Could you check a few things on this drawing? It's one solid part, dimensions in mm from its lowest x, y, z. Coordinates: 2 decimals unless noted, no trailing zeros. Order: outer loops, then holes, each group sorted by start corner. A loop starts at its lowest first (then second) coordinate and runs counter-clockwise, first axis right, second up.
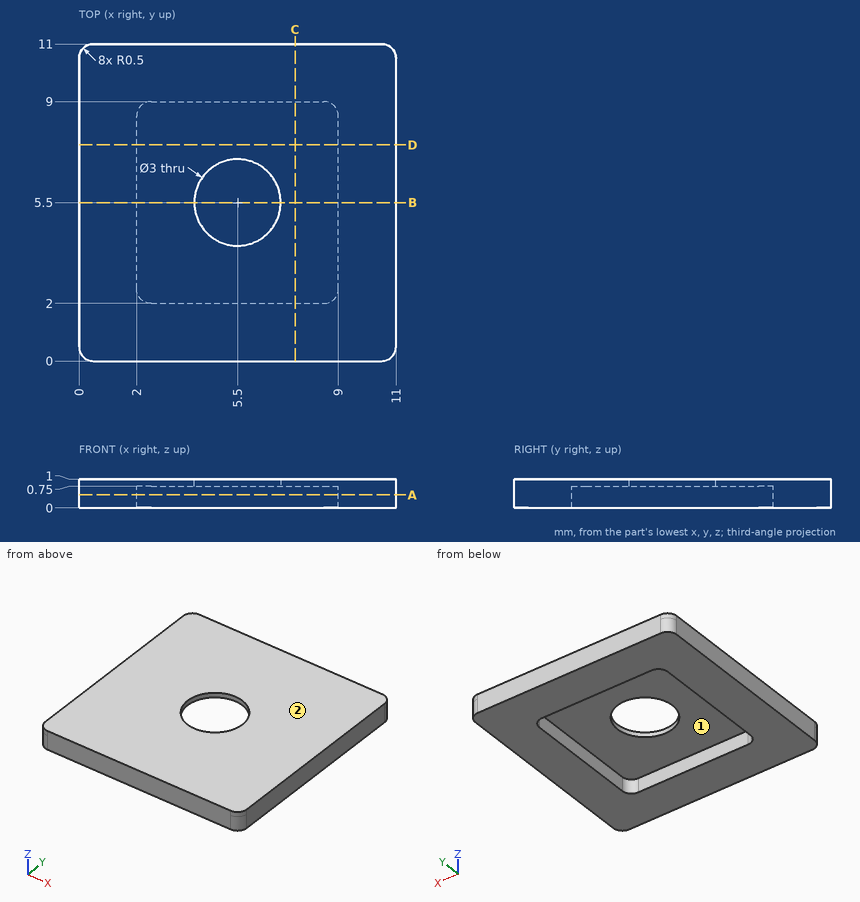
1. Imagine slicing it at C-C on x = 7.5. Please give me the cut outline in (y, z), then the cut area to 3 significant figures.
Completed:
outline: (0, 0) - (2, 0) - (2, 0.75) - (9, 0.75) - (9, 0) - (11, 0) - (11, 1) - (0, 1) - close
area: 5.75 mm2
2. Imagine slicing it at B-B on y = 5.5. Please give me the cut outline in (x, z), then the cut area to 3 significant figures.
Completed:
outline: (0, 0) - (2, 0) - (2, 0.75) - (4, 0.75) - (4, 1) - (0, 1) - close; (7, 0.75) - (9, 0.75) - (9, 0) - (11, 0) - (11, 1) - (7, 1) - close
area: 5.00 mm2
3. Please list where these lines run through material, in increasing order: probe 1 along Y at (x, z) = (8, 0.25); probe 2 along Y at (x, z) = (5.5, 0.9).
Completed:
probe 1: y = 0 to 2, 9 to 11
probe 2: y = 0 to 4, 7 to 11
4. Thinking about a two-plate mould opening in X: for the marked faces 1 and 2, which applies, pulls with the +X half, pulls with the -X half, needs draft (parallel to the pull), parting line crosses it, or undercut?
Completed:
face 1: undercut
face 2: needs draft
5. Imagine slicing it at A-A on z = 0.45. Please give me the cut outline in (x, y).
Completed:
outline: (0, 0.5) arc R0.5 ccw to (0.5, 0) - (10.5, 0) arc R0.5 ccw to (11, 0.5) - (11, 10.5) arc R0.5 ccw to (10.5, 11) - (0.5, 11) arc R0.5 ccw to (0, 10.5) - close; hole (2, 2.5) arc R0.5 ccw to (2.5, 2) - (8.5, 2) arc R0.5 ccw to (9, 2.5) - (9, 8.5) arc R0.5 ccw to (8.5, 9) - (2.5, 9) arc R0.5 ccw to (2, 8.5) - close
6. I'm going to push a flat-ended pin straight in: pin 1 (5 mm diameter, centred on x = 5.5, y = 5.5, fed in from -Z). Where does the tip first touch, or does it pass through?
Completed:
pin 1: stops at z = 0.75
